Here's the drawing with two shaded views (mm, measured from the low corner). I have some questions. Give positions to 0.01 mm unless a question says otherwise; leave off trailing zeros. Order: outer loops, then holes, each group sorted by start corner. A loop starts at its lowest first (then second) coordinate and runs counter-clockwise, first axis right, second up. Notation, with made-up numbers: M -19,36.25 L -8,36.25 A21 cw -8,60.25 Z; hole C -6.5,-14.75 d4. An arc over 180 degrees is marked long. Use a Markdown table: item, result. Add a question column.
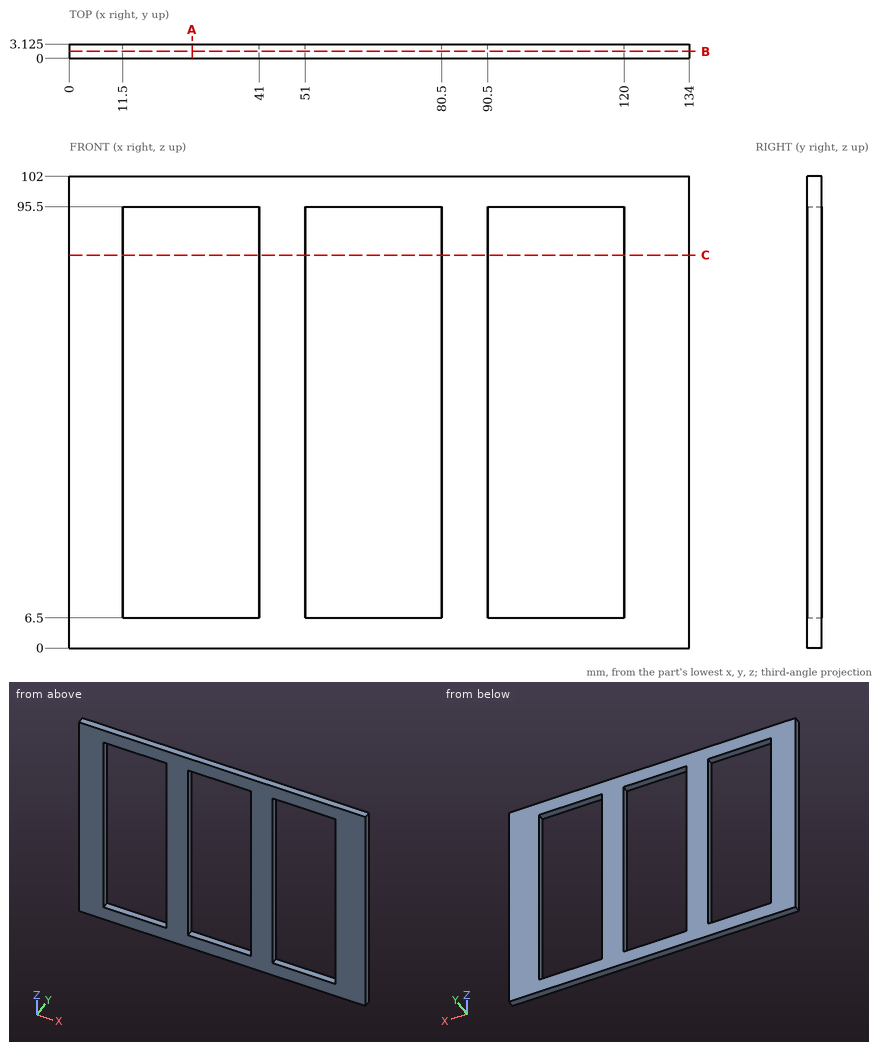
1) Suppose I cut it at B-B on y = 1.55. Please give me the cut outline in (x, z), and give its area (3 significant figures).
2) Please list where these lines run through material, in increasing order: line 1 (X direction, y = 1.4, z = 20); line 2 (Z direction, x = 112.5, y = 0.6). Write a range as from..to.
3) Suppose I cut it at C-C on z = 85. Please give me the cut outline in (x, y) (3 decimals), and give its area (3 significant figures).
4) Suppose I cut it at A-A on x = 26.5. Please give me the cut outline in (y, z) (3 decimals), and give its area (3 significant figures).
Values found:
| question | item | result |
|---|---|---|
| 1 | outline | M 0,0 L 134,0 L 134,102 L 0,102 Z; hole M 11.5,6.5 L 41,6.5 L 41,95.5 L 11.5,95.5 Z; hole M 51,6.5 L 80.5,6.5 L 80.5,95.5 L 51,95.5 Z; hole M 90.5,6.5 L 120,6.5 L 120,95.5 L 90.5,95.5 Z |
| 1 | area | 5,790 mm^2 |
| 2 | line 1 | x = 0..11.5, 41..51, 80.5..90.5, 120..134 |
| 2 | line 2 | z = 0..6.5, 95.5..102 |
| 3 | outline | M 0,0 L 11.5,0 L 11.5,3.125 L 0,3.125 Z; M 41,0 L 51,0 L 51,3.125 L 41,3.125 Z; M 80.5,0 L 90.5,0 L 90.5,3.125 L 80.5,3.125 Z; M 120,0 L 134,0 L 134,3.125 L 120,3.125 Z |
| 3 | area | 142 mm^2 |
| 4 | outline | M 0,0 L 3.125,0 L 3.125,6.5 L 0,6.5 Z; M 0,95.5 L 3.125,95.5 L 3.125,102 L 0,102 Z |
| 4 | area | 40.6 mm^2 |
